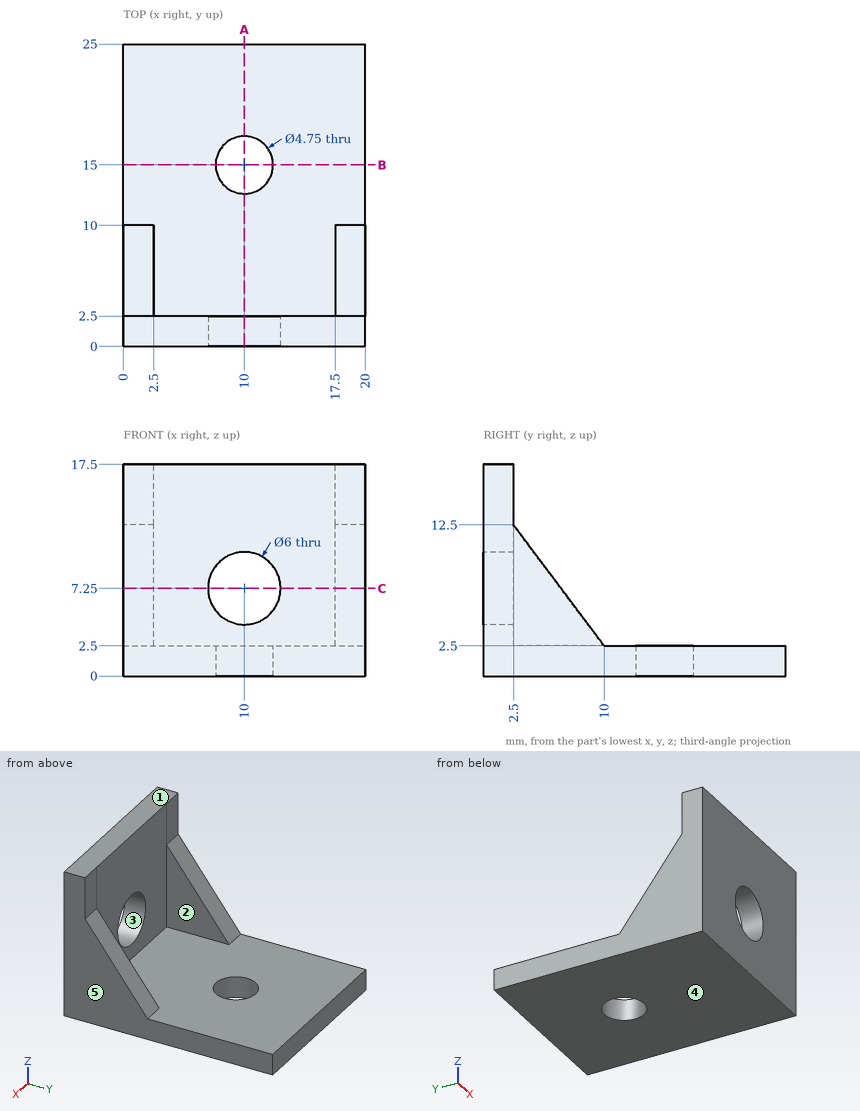
Can you work these out from the drawing? Everything is in mm from the part's minimum corner. A direction names the side the tool comes from. Coordinates: 2 decimals unless noted, no trailing zeros. Loops run counter-clockwise (first coordinate to the right, second up) from the corner with the lowest first, then second, coordinate; pieces in that order, holes last. Notation, with made-up numbers: (86.25, 29.25) - (100.25, 29.25) arc R14 cw to (100.25, 45.25) - close; hole circle Ø9 at (30.25, 20.5). An arc over 180 degrees is marked (long way). Put each result on its own line as item: value. Start each with the question number.
Item 1: If I drill on line 1 along X through (y, z) = (4.5, 6.5); line 2 along Z through (x, y) = (4.5, 10), over which ranges is the centre line in solid material (lowest first)?
Item 2: Suppose I cut it at C-C (z = 7.25). Please give me the cut outline in (x, y), and give its area (3 significant figures).
Item 3: Which directions (+Z, -Z, +X, -X, +Y, -Y) give clear straight access to the entire face, cutting with the end or side of a thin tool? Please do the marked faces 1 and 2.
Item 4: Suppose I cut it at A-A (x = 10). Please give me the cut outline in (y, z) (3 decimals).
Item 5: If we mould it in two halves opening along Z, with no side actions, what happens to the marked faces 3, 4 and 5? For each: +Z half, -Z half, draft (parallel to the pull), parting line (faces both ways), or undercut.
Item 6: For pin 1 (6 mm diameter, centred on x = 12.5, y = 16.5, fed in from +Z); pin 2 (4 mm diameter, centred on x = 3, z = 13.5, fed in from +Y); pin 3 (2 mm diameter, centred on x = 0.5, z = 14.5, fed in from +Y), each with a flat end and sliding along its axis, tell me the tip position at first contact or that it passes through.
Item 7: Suppose I cut it at B-B (y = 15). Please give me the cut outline in (x, z) (3 decimals).
Here are the results:
1. line 1: 0 to 2.5, 17.5 to 20
1. line 2: 0 to 2.5
2. outline: (0, 0) - (7, 0) - (7, 2.5) - (2.5, 2.5) - (2.5, 6.44) - (0, 6.44) - close; (13, 0) - (20, 0) - (20, 6.44) - (17.5, 6.44) - (17.5, 2.5) - (13, 2.5) - close
2. area: 54.7 mm²
3. face 1: +Z, +X, -X, +Y, -Y
3. face 2: +Z, +Y
4. outline: (0, 0) - (12.625, 0) - (12.625, 2.5) - (2.5, 2.5) - (2.5, 4.25) - (0, 4.25) - close; (0, 10.25) - (2.5, 10.25) - (2.5, 17.5) - (0, 17.5) - close; (17.375, 0) - (25, 0) - (25, 2.5) - (17.375, 2.5) - close
5. face 3: undercut
5. face 4: -Z half
5. face 5: draft
6. pin 1: z = 2.5
6. pin 2: y = 3.2
6. pin 3: y = 2.5
7. outline: (0, 0) - (7.625, 0) - (7.625, 2.5) - (0, 2.5) - close; (12.375, 0) - (20, 0) - (20, 2.5) - (12.375, 2.5) - close
